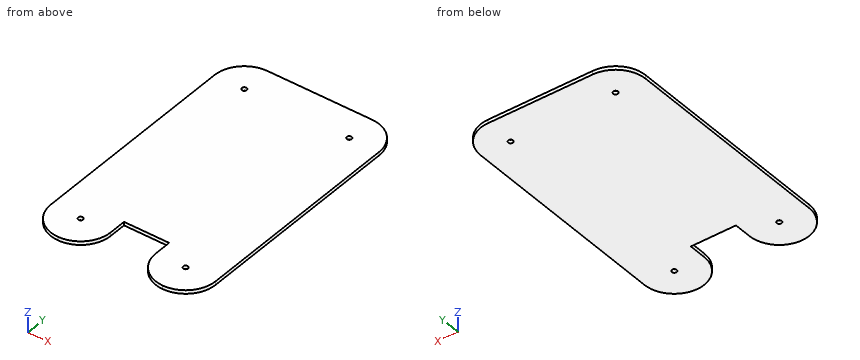
```python
from build123d import *

# Parameters (mm, degrees)
F0_R     = 2.75
F1_DEPTH = 4
F2_W     = 287.6251339912
F2_H     = 352.3535430431
F3_DEPTH = 25
F5_DEPTH = 25


with BuildPart() as f1:
    # F0 (on Top) → F1 (new body)
    with BuildSketch(Plane.XY):
        with BuildLine():
            ThreePointArc((92.7, 122.49998), (83.576376234, 144.526356234), (61.55, 153.64998))
            Line((61.55, 153.64998), (-61.55, 153.64998))
            ThreePointArc((-61.55, 153.64998), (-83.576376234, 144.526356234), (-92.7, 122.49998))
            Line((-92.7, 122.49998), (-92.7, -122.49998))
            ThreePointArc((-92.7, -122.49998), (-83.576376234, -144.526356234), (-61.55, -153.64998))
            Line((-61.55, -153.64998), (61.55, -153.64998))
            ThreePointArc((61.55, -153.64998), (83.576376234, -144.526356234), (92.7, -122.49998))
            Line((92.7, -122.49998), (92.7, 122.49998))
        make_face()
        with Locations((-59.05, -119.99998)):
            Circle(F0_R, mode=Mode.SUBTRACT)
        with Locations((59.05, -119.99998)):
            Circle(F0_R, mode=Mode.SUBTRACT)
        with Locations((-59.05, 119.99998)):
            Circle(F0_R, mode=Mode.SUBTRACT)
        with Locations((59.05, 119.99998)):
            Circle(F0_R, mode=Mode.SUBTRACT)
    extrude(amount=F1_DEPTH)

    # F2 (on face) → F3 (cut)
    with BuildSketch(Plane.XY.offset(4)):
        Rectangle(F2_W, F2_H)
        with BuildLine():
            ThreePointArc((-92.7, 119.99998), (-82.8441431869, 143.7941231869), (-59.05, 153.64998))
            Line((-59.05, 153.64998), (59.05, 153.64998))
            ThreePointArc((59.05, 153.64998), (82.8441431869, 143.7941231869), (92.7, 119.99998))
            Line((92.7, 119.99998), (92.7, -119.99998))
            ThreePointArc((92.7, -119.99998), (82.8441431869, -143.7941231869), (59.05, -153.64998))
            Line((59.05, -153.64998), (-59.05, -153.64998))
            ThreePointArc((-59.05, -153.64998), (-82.8441431869, -143.7941231869), (-92.7, -119.99998))
            Line((-92.7, -119.99998), (-92.7, 119.99998))
        make_face(mode=Mode.SUBTRACT)
    extrude(amount=-F3_DEPTH, mode=Mode.SUBTRACT)

    # F4 (on face) → F5 (cut)
    with BuildSketch(Plane.XY.offset(4)):
        with BuildLine():
            ThreePointArc((59.05, -153.64998), (35.2558568131, -143.7941231869), (25.4, -119.99998))
            Line((25.4, -119.99998), (25.4, -100.35002))
            Line((25.4, -100.35002), (0, -100.35002))
            Line((0, -100.35002), (-25.4, -100.35002))
            Line((-25.4, -100.35002), (-25.4, -119.99998))
            ThreePointArc((-25.4, -119.99998), (-35.2558568131, -143.7941231869), (-59.05, -153.64998))
            Line((-59.05, -153.64998), (59.05, -153.64998))
        make_face()
    extrude(amount=-F5_DEPTH, mode=Mode.SUBTRACT)


solid = f1.part
```
For this review, take the finished solid that the model builds, in its own axes (mm). Give positions to 0.01 mm unless a question says otherwise; leave off trailing zeros. Order: outer loops, then holes, each group sorted by start corner. A loop starts at its lowest first (then second) coordinate and runs counter-clockwise, first axis right, second up.
1) Take a section at C-C (x = -12.5). Give the boundary of the cut face in (y, z).
2) Take a section at D-D (y = 131.5). Give the boundary of the cut face in (x, z).
3) Wall thickness on line 1 (Y direction, x = 59.05, z = 1.7); line 2 (X direction, y = 121, z = 2.65); line 3 (Y direction, x = -15, z = 2.2): over which ranges is each line inside the solid? List them lowest first.
4) Take a section at A-A (z = 2.4). Give the boundary of the cut face in (x, y).
5) Insertion check: pin 1 (3.5 mm diameter, centred on x = 59.05, y = -120, fed in from +Z); pin 2 (1 mm diameter, centred on x = -4.5, z = 0.5, fed in from -Y); pin 3 (1.5 mm diameter, centred on x = 63.5, z = 3, fed in from -Y). Each pin has a flat end and moves straight along its axis. Give the tip position at first contact, or say it passes through.
6) Take a section at B-B (y = -132). Give the boundary of the cut face in (x, z), then the cut area to 3 significant figures.
Derived:
1. outline: (-100.35, 0) - (153.65, 0) - (153.65, 4) - (-100.35, 4) - close
2. outline: (-90.67, 0) - (90.67, 0) - (90.67, 4) - (-90.67, 4) - close
3. line 1: y = -153.65 to -122.75, -117.25 to 117.25, 122.75 to 153.65
3. line 2: x = -92.69 to -61.61, -56.49 to 56.49, 61.61 to 92.69
3. line 3: y = -100.35 to 153.65
4. outline: (-92.7, -120) arc R33.65 ccw to (-25.4, -120) - (-25.4, -100.35) - (25.4, -100.35) - (25.4, -120) arc R33.65 ccw to (92.7, -120) - (92.7, 120) arc R33.65 ccw to (59.05, 153.65) - (-59.05, 153.65) arc R33.65 ccw to (-92.7, 120) - close; hole circle Ø5.5 at (-59.05, -120); hole circle Ø5.5 at (-59.05, 120); hole circle Ø5.5 at (59.05, -120); hole circle Ø5.5 at (59.05, 120)
5. pin 1: passes through
5. pin 2: stops at y = -100.35
5. pin 3: stops at y = -153.45
6. outline: (-90.49, 0) - (-27.61, 0) - (-27.61, 4) - (-90.49, 4) - close; (27.61, 0) - (90.49, 0) - (90.49, 4) - (27.61, 4) - close
6. area: 503 mm2
